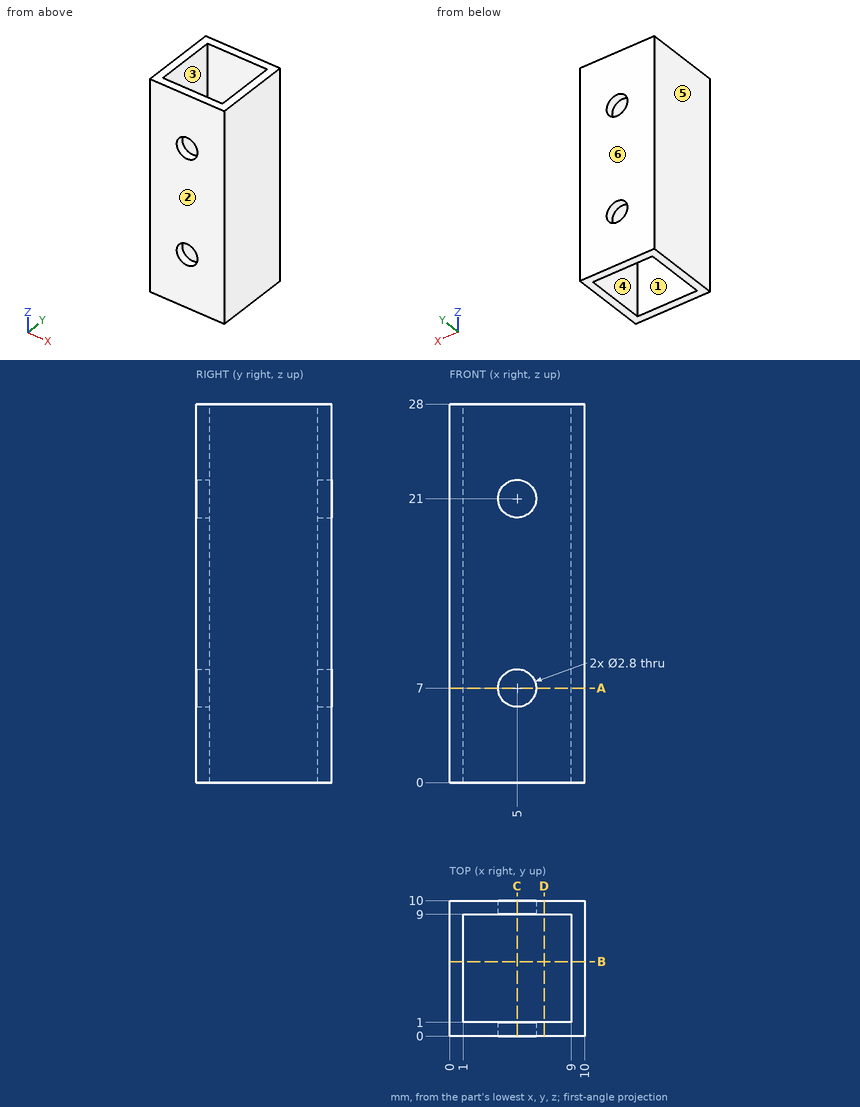
Source: three-view drawing plus pictorial views. Frame: mm from the lowest corner of the part. A direction names the side the tool comes from. Round coordinates to 2 decimals unless told otherwise and drop trailing zeros. Loops run counter-clockwise (first coordinate to the right, second up) from the corner with the lowest first, then second, coordinate; pieces in that order, holes last. Notation, with made-up numbers: M 49,87 L 104,87 A8 ccw 104,94 Z; hole C 10.25,36 d7. An arc over 180 degrees is marked long. Put each result on its own line as item: value.
(1) Pull-direction query (X, two-part tool) for the marked faces 3, 4, 5 and 6; classes: released by +X, released by -X, zero draft, split by the parting line, or undercut.
Solutions:
face 3: undercut
face 4: undercut
face 5: released by -X
face 6: zero draft
(2) Access query for the marked faces 1 and 2. Directions: +Z, -Z, +X, -X, +Y, -Y. A direction counts if a zero-diameter tool reaches every point of the face in a straight line with its end or side. Return the directions, or none.
Solutions:
face 1: +Z, -Z
face 2: +Z, -Z, +X, -X, -Y
(3) Ray query, line 1 (Z direction, x = 5, y = 9.85); line 2 (X direction, y = 5, z = 13.5). Return the intervals inside material, ascending. Write a range as [from, to].
Solutions:
line 1: [0, 5.6], [8.4, 19.6], [22.4, 28]
line 2: [0, 1], [9, 10]
(4) Section C-C, the plane x = 5. Return loops of the section in (y, z).
Solutions:
outline: M 0,0 L 1,0 L 1,5.6 L 0,5.6 Z; M 0,8.4 L 1,8.4 L 1,19.6 L 0,19.6 Z; M 0,22.4 L 1,22.4 L 1,28 L 0,28 Z; M 9,0 L 10,0 L 10,5.6 L 9,5.6 Z; M 9,8.4 L 10,8.4 L 10,19.6 L 9,19.6 Z; M 9,22.4 L 10,22.4 L 10,28 L 9,28 Z
(5) Section B-B, the plane y = 5.5. Return loops of the section in (x, z), and give its area (3 significant figures).
Solutions:
outline: M 0,0 L 1,0 L 1,28 L 0,28 Z; M 9,0 L 10,0 L 10,28 L 9,28 Z
area: 56.0 mm²
(6) First-contact query: pin 1 (1.7 mm diameter, centred on x = 5, z = 21, fed in from -Y). Flat tip, straight axial feed; report the tip coordinate or a pass-through.
Solutions:
pin 1: through
(7) Section A-A, the plane z = 7. Return loops of the section in (x, y), and give its area (3 significant figures).
Solutions:
outline: M 0,0 L 3.6,0 L 3.6,1 L 1,1 L 1,9 L 3.6,9 L 3.6,10 L 0,10 Z; M 6.4,0 L 10,0 L 10,10 L 6.4,10 L 6.4,9 L 9,9 L 9,1 L 6.4,1 Z
area: 30.4 mm²
